Input: part model. Units: mm. Frame: model coordinates. Face numbers are marked on the shaded views. A direction names the side the tool comes from. Give positions to 0.01 mm unless a question says otherwise; leave off trailing zeros. Loops run counter-clockwise (first coordinate to the right, second up) from the corner with the lowest first, then second, coordinate; pieces in that order, holes last. Notation, with made-up numbers: (26, 49.25) -> (67, 49.25) arc R17 ccw to (67, 66.25) -> close; hole circle Ø5 at (3.25, 24.25). An arc over 180 degrees is marked (long way). One line per question, with ' | ' between items.
from build123d import *

# Parameters (mm, degrees)
SKETCH1_R                = 15
BOSS_EXTRUDE1_DEPTH      = 15
SKETCH2_R                = 1.5
BOSS_EXTRUDE2_DEPTH      = 4
BOSS_EXTRUDE3_DEPTH      = 0.5
BOSS_EXTRUDE3_DEPTH_BACK = 4.5
SKETCH3_R                = 3.75
SKETCH3_R_2              = 1.5
FILLET1_R                = 1


with BuildPart() as part:
    # Sketch1 → Boss-Extrude1 (new body)
    with BuildSketch(Plane(origin=(0, 0, 0), x_dir=(1, 0, 0), z_dir=(0, 1, 0))):
        with Locations(Location((0, 0, 0), (0, 0, 270))):
            Circle(SKETCH1_R)
    extrude(amount=BOSS_EXTRUDE1_DEPTH)

    # Sketch2 → Boss-Extrude2 (add)
    # profile 1 of 2: a face of its own
    with BuildSketch(Plane(origin=(0, 0, 0), x_dir=(1, 0, 0), z_dir=(0, 1, 0))):
        with BuildLine():
            ThreePointArc((-8.333333333, 12.472191289), (-15, 0), (-8.333333333, -12.472191289))
            Line((-8.333333333, -12.472191289), (-22.333333333, -3.118047822))
            ThreePointArc((-22.333333333, -3.118047822), (-24, 0), (-22.333333333, 3.118047822))
            Line((-22.333333333, 3.118047822), (-8.333333333, 12.472191289))
        make_face()
        with Locations(Location((-20.25, 0, 0), (0, 0, 270))):
            Circle(SKETCH2_R, mode=Mode.SUBTRACT)
    # profile 2 of 2: a face of its own
    with BuildSketch(Plane(origin=(0, 0, 0), x_dir=(1, 0, 0), z_dir=(0, 1, 0))):
        with BuildLine():
            Line((8.333333333, 12.472191289), (22.333333333, 3.118047822))
            ThreePointArc((22.333333333, 3.118047822), (24, 0), (22.333333333, -3.118047822))
            Line((22.333333333, -3.118047822), (8.333333333, -12.472191289))
            ThreePointArc((8.333333333, -12.472191289), (15, 0), (8.333333333, 12.472191289))
        make_face()
        with Locations(Location((20.25, 0, 0), (0, 0, 270))):
            Circle(SKETCH2_R, mode=Mode.SUBTRACT)
    extrude(amount=BOSS_EXTRUDE2_DEPTH)

    # Sketch3 → Boss-Extrude3 (add, two sides: drawn at the far end of the back side and taken through both)
    # profile 1 of 2: a face of its own
    with BuildSketch(Plane(origin=(0, 4, 0), x_dir=(1, 0, 0), z_dir=(0, 1, 0)).offset(-BOSS_EXTRUDE3_DEPTH_BACK)):
        with Locations(Location((-20.25, 0, 0), (0, 0, 270))):
            Circle(SKETCH3_R)
        with Locations(Location((-20.25, 0, 0), (0, 0, 270))):
            Circle(SKETCH3_R_2, mode=Mode.SUBTRACT)
    # profile 2 of 2: a face of its own
    with BuildSketch(Plane(origin=(0, 4, 0), x_dir=(1, 0, 0), z_dir=(0, 1, 0)).offset(-BOSS_EXTRUDE3_DEPTH_BACK)):
        with Locations(Location((20.25, 0, 0), (0, 0, 270))):
            Circle(SKETCH3_R)
        with Locations(Location((20.25, 0, 0), (0, 0, 270))):
            Circle(SKETCH3_R_2, mode=Mode.SUBTRACT)
    extrude(amount=BOSS_EXTRUDE3_DEPTH + BOSS_EXTRUDE3_DEPTH_BACK)

    # Fillet1
    fillet1_edges = [part.edges().sort_by_distance(p)[0] for p in [
        (0, 15, -15),
    ]]
    fillet(fillet1_edges, radius=FILLET1_R)


solid = part.part
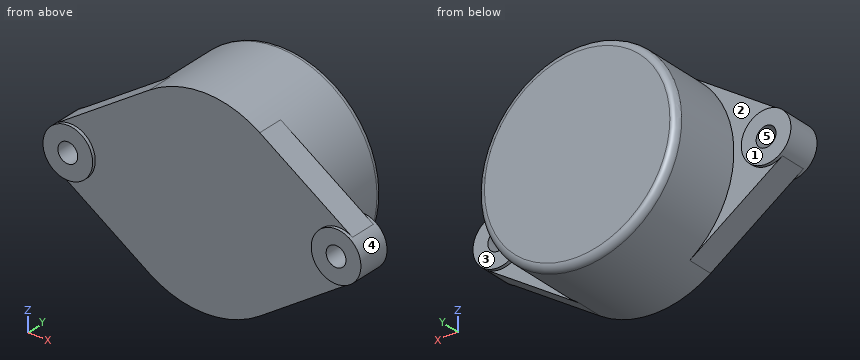
1. Section query C-C (y = 8.5). Output: boundary loops of the cut face in (x, z).
Determined:
outline: circle Ø30 at (0, 0)
2. Pin query (flat end, axial travel): P1, Ø7, axis at x = -18, z = -5.5, coming from the +Y side; P2, Ø6, axis at x = -18.5, y = 2, coming from the -Z side; P3, Ø8, axis at x = -8, y = 9.5, coming from the +Z side; P4, Ø1, axis at x = 13.5, z = 5, coming from the +Y side. Return the tip coordinate at first contact, or that it passes through.
Determined:
P1: stops at y = 4.5 | P2: stops at z = -7.68 | P3: stops at z = 14.46 | P4: stops at y = 15
3. Section query A-A (x = 20.25). Output: boundary loops of the cut face in (y, z).
Determined:
outline: (-0.5, -3.75) -> (0, -3.75) -> (0, -4.51) -> (4, -4.51) -> (4, -3.75) -> (4.5, -3.75) -> (4.5, -1.5) -> (-0.5, -1.5) -> close; (-0.5, 1.5) -> (4.5, 1.5) -> (4.5, 3.75) -> (4, 3.75) -> (4, 4.51) -> (0, 4.51) -> (0, 3.75) -> (-0.5, 3.75) -> close
4. Reachability of the marked faces 1, 2, 3, 4 and 5 from +Z, -Z, +X, -X, +Y, -Y: full face, straight path, thin tool, end or side. Return the list, or none.
Determined:
face 1: +Z, -Z, -X, +Y | face 2: +Y | face 3: +Z, -Z, +X, +Y | face 4: none | face 5: +Y, -Y
5. Section query B-B (x = 0). Output: boundary loops of the cut face in (y, z).
Determined:
outline: (0, -15) -> (14, -15) arc R1 ccw to (15, -14) -> (15, 14) arc R1 ccw to (14, 15) -> (0, 15) -> close
6. Ray query, line 1 along X through (y, z) = (1.45, 0); line 2 along Y through (x, z) = (-5.5, 11.25); line 3 along Y through (x, z) = (-21, 2). Return the intervals inside material, ascending. Write a range as from..to.
Determined:
line 1: x = -24..-21.75, -18.75..18.75, 21.75..24 | line 2: y = 0..15 | line 3: y = -0.5..4.5
